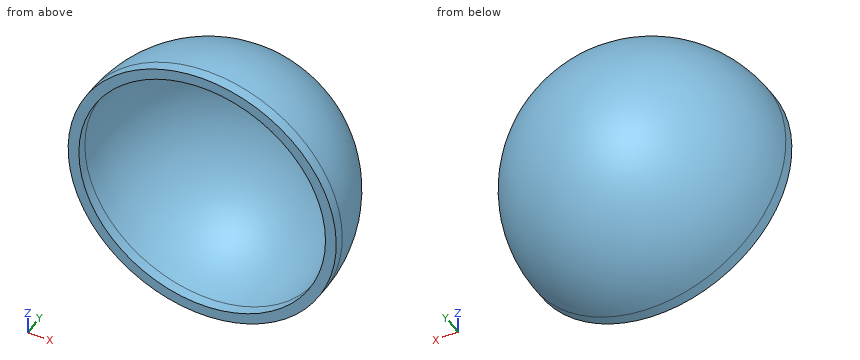
```python
from build123d import *

# Parameters (mm, degrees)
SKETCH1_R           = 25
BOSS_EXTRUDE1_DEPTH = 2
DOME1_FACE_RADIUS   = 25
DOME1_HEIGHT        = 25


# Read off the part's stored shape, not the designer's step: Shell1
with BuildPart() as part:
    # Sketch1 → Boss-Extrude1 (new body)
    with BuildSketch(Plane(origin=(0, 0, 0), x_dir=(1, 0, 0), z_dir=(0, 1, 0))):
        with Locations(Location((0, 0, 0), (0, 0, 270))):
            Circle(SKETCH1_R)
    extrude(amount=BOSS_EXTRUDE1_DEPTH)

    # Dome1: a dome of height H over a round flat face of radius A is a cap of a sphere of radius (A * A + H * H) / (2 * H)
    dome1_r = (DOME1_FACE_RADIUS * DOME1_FACE_RADIUS + DOME1_HEIGHT * DOME1_HEIGHT) / (2 * DOME1_HEIGHT)
    dome1_base = Plane((0, 2, 0), z_dir=(0, 1, 0))
    with Locations(dome1_base.offset(DOME1_HEIGHT - dome1_r)):
        dome1_ball = Sphere(dome1_r, mode=Mode.PRIVATE)
    add(split(dome1_ball, bisect_by=dome1_base, keep=Keep.TOP, mode=Mode.PRIVATE))

    # Shell1 outline → Shell1 (revolve, cut)
    with BuildSketch(Plane.XY):
        with BuildLine():
            Line((23, 0), (23, 1.999999977))
            ThreePointArc((23, 1.999999977), (16.263455975, 18.263455959), (0, 25))
            Line((0, 25), (0, 0))
            Line((0, 0), (23, 0))
        make_face()
    revolve(axis=Axis((0, 0, 0), (0, 1, 0)), mode=Mode.SUBTRACT)


solid = part.part
```
For this review, take the finished solid that the model builds, in its own axes (mm). Round coordinates to 2 decimals unless told otherwise and drop trailing zeros. Loops run counter-clockwise (first coordinate to the right, second up) from the corner with the lowest first, then second, coordinate; pieces in that order, holes last.
(1) We need section B-B (z = 0). Give the boundary of the cut face in (x, y).
Returned:
outline: (-25, 0) - (-23, 0) - (-23, 2) arc R23 cw to (23, 2) - (23, 0) - (25, 0) - (25, 2) arc R25 ccw to (-25, 2) - close
(2) We need section A-A (x = 0). Give the boundary of the cut face in (y, z), plus the area to 3 significant figures.
Returned:
outline: (0, -25) - (2, -25) arc R25 ccw to (2, 25) - (0, 25) - (0, 23) - (2, 23) arc R23 cw to (2, -23) - (0, -23) - close
area: 159 mm2
(3) Wall thickness on line 1 along X through (y, z) = (0.4, 0); line 2 along X through (y, z) = (12.25, 10.5); line 3 along Z through (x, y) = (-14, 17.5): over which ranges is each line inside the solid? List them lowest first.
Returned:
line 1: x = -25 to -23, 23 to 25
line 2: x = -20.24 to -17.71, 17.71 to 20.24
line 3: z = -13.74 to -9.63, 9.63 to 13.74
(4) Clearance check with flat-ended pins moving along their axes: P1, Ø10, axis at x = 13.5, y = 13, coming from the -Z side; P2, Ø3, axis at x = -7.5, y = 4, coming from the -Z side; P3, Ø1, axis at x = 3.5, y = 4.5, coming from the -Z side. State where each tip first meets the part, or that it passes through.
Returned:
P1: stops at z = -21.7
P2: stops at z = -24.2
P3: stops at z = -24.71
(5) We need section C-C (y = 11). Give the boundary of the cut face in (x, z).
Returned:
outline: circle Ø46.65 at (0, 0); hole circle Ø42.33 at (0, 0)
